Check sheet for the drawn part. Datum: minimum x, y, z corner. Units: mm. A direction names the side the tool comes from. Coordinates: 2 decimals unless noted, no trailing zeros. Loops run counter-clockwise (first coordinate to the right, second up) from the corner with the lowest first, then second, coordinate; pieces in that order, holes last. Notation, with made-up numbers: (62, -39.5) - (77, -39.5) arc R20 ccw to (77, -1.5) - close; hole circle Ø6 at (3, 19). An arc over 180 degrees is marked (long way). Answer as a JSON object with one key per item and string values. Group by question number.
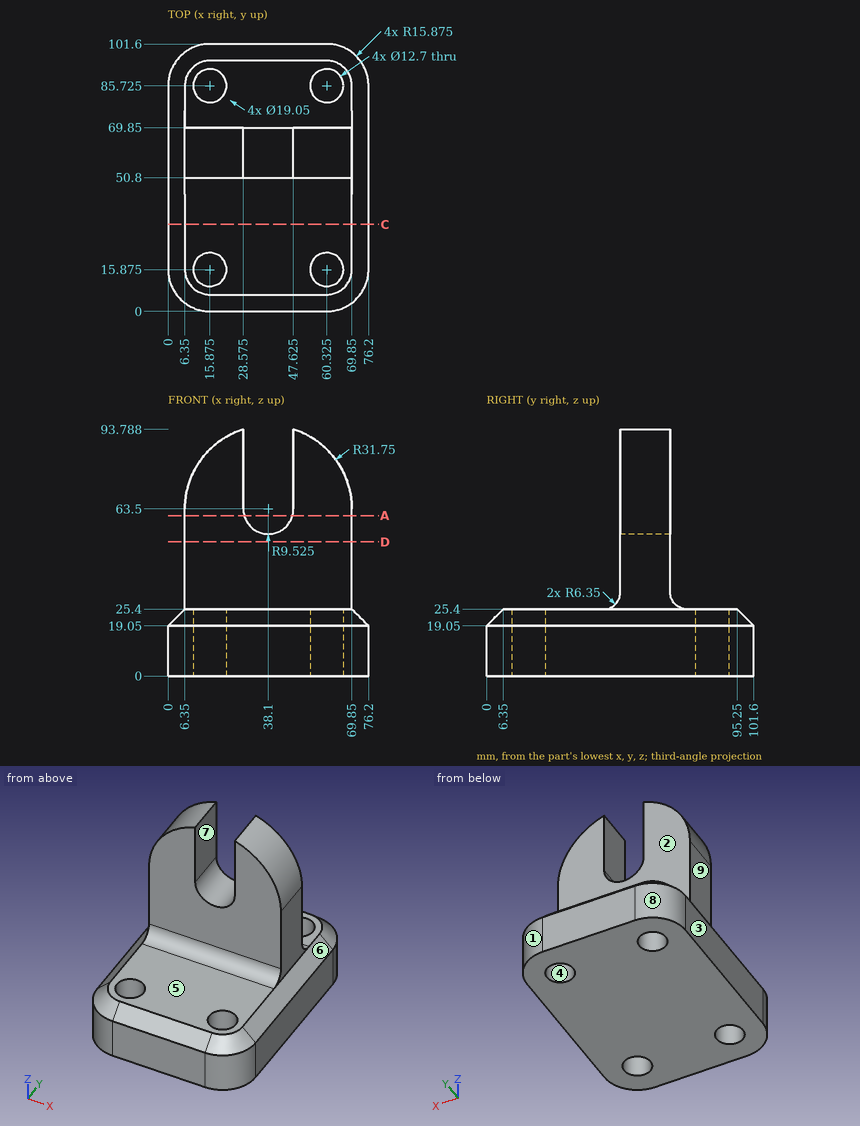
1. Sectioned sample at D-D on z = 51. Record the cut outline in (x, y), plus the area to 3 significant figures.
2. Release check for a two-part mould opening along X. For the marked faces 1, 2, 3 and 4 record: released by +X, released by -X, zero draft, split by the parting line, or undercut.
3. Gauge pin test, flat ends, axial feed: pin 1 (16 mm diameter, centred on y = 66.5, z = 50, fed in from +X); pin 2 (16.5 mm diameter, centred on x = 15.875, y = 15.875, fed in from -Z); pin 3 (8 mm diameter, centred on y = 54, z = 28, fed in from -X); pin 4 (1.5 mm diameter, centred on x = 67.5, y = 20.5, fed in from +Z). Record the tip position at first contact, or that the pin passes through.
4. Access from +Z, -Z, +X, -X, +Y, -Y to the whole of each face (thin tool, end or side, straight path). Record for the marked faces 5, 6, 7, 8 and 9.
5. Material ranges on line 1 (X direction, y = 10.5, z = 6) (1 decimal); line 2 (Y direction, x = 55, z = 6.5) (1 decimal); line 3 (Z direction, x = 37, y = 25), recorded low to high.
6. Sectioned sample at A-A on z = 61. Record the cut outline in (x, y).
7. Sectioned sample at C-C on y = 33. Record the cut outline in (x, z).
Answers follow:
{
 "1": {"outline": "(6.35, 50.8) - (69.85, 50.8) - (69.85, 69.85) - (6.35, 69.85) - close", "area": "1,210 mm^2"},
 "2": {"face 1": "released by +X", "face 2": "zero draft", "face 3": "released by -X", "face 4": "undercut"},
 "3": {"pin 1": "stops at x = 69.85", "pin 2": "stops at z = 0", "pin 3": "stops at x = 4.95", "pin 4": "stops at z = 25.4"},
 "4": {"face 5": "+Z, +X, -X, -Y", "face 6": "+Z, +X, +Y, -Y", "face 7": "+Z, +Y, -Y", "face 8": "+Z, -Z, -X, +Y", "face 9": "+Z, -X, +Y, -Y"},
 "5": {"line 1": "x = 0.9 to 12.5, 19.3 to 56.9, 63.7 to 75.3", "line 2": "y = 0 to 12.4, 19.3 to 82.3, 89.2 to 101.6", "line 3": "z = 0 to 25.4"},
 "6": {"outline": "(6.35, 50.8) - (28.91, 50.8) - (28.91, 69.85) - (6.35, 69.85) - close; (47.29, 50.8) - (69.85, 50.8) - (69.85, 69.85) - (47.29, 69.85) - close"},
 "7": {"outline": "(0, 0) - (76.2, 0) - (76.2, 19.05) - (69.85, 25.4) - (6.35, 25.4) - (0, 19.05) - close"}
}
